Design review of the part built by this model. Coordinates are the model's own, in mm. Face numbers are marked on the shaded views. A direction names the side the tool comes from. Coordinates: 2 decimals unless noted, no trailing zeros. Order: outer loops, then holes, each group sorted by start corner. A loop starts at its lowest first (then second) coordinate and runs counter-clockwise, first axis right, second up. Notation, with made-up numbers: M 37.5,50 L 48.5,50 A23 ccw 48.5,76 Z; hole C 81.5,77 d7. An arc over 180 degrees is marked long. Answer as a JSON object with one key per item and string values.
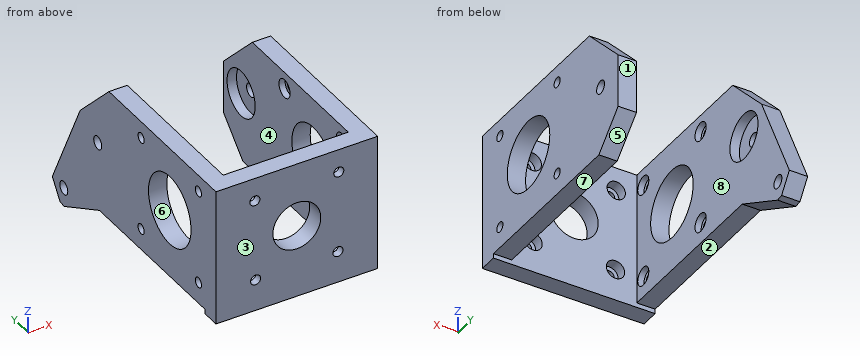
from build123d import *

# Parameters (mm, degrees)
EXTRUDE_1_DEPTH     = 64
SKETCH_2_R          = 7.85
SKETCH_2_R_2        = 1.65
CUT_EXTRUDE_1_DEPTH = 20
SKETCH_3_R          = 3
CUT_EXTRUDE_2_DEPTH = 3.5
CUT_EXTRUDE_3_DEPTH = 111.938045773
SKETCH_5_R          = 11.5
SKETCH_5_R_2        = 1.65
SKETCH_5_R_3        = 2.15
CUT_EXTRUDE_4_DEPTH = 104.981969591
SKETCH_6_R          = 7.6
CUT_EXTRUDE_5_DEPTH = 3.1
CUT_EXTRUDE_START   = -3.1
SKETCH_7_R          = 7.6
CUT_EXTRUDE_6_DEPTH = 3.1
SKETCH_10_R         = 2.15
EXTRUDE_3_DEPTH     = 6
SKETCH_11_R         = 3
CUT_EXTRUDE_7_DEPTH = 2
CUT_EXTRUDE_START_2 = -2
SKETCH_12_R         = 3
CUT_EXTRUDE_8_DEPTH = 2


with BuildPart() as part:
    # 草图1 → 凸台-拉伸1 (new body)
    with BuildSketch(Plane.XY):
        Polygon((-20.5, 73.5), (-26.5, 73.5), (-26.5, 0), (26.5, 0), (26.5, 73.5), (20.5, 73.5), (20.5, 6), (-20.5, 6), align=None)
    extrude(amount=EXTRUDE_1_DEPTH)

    # 草图2 → 切除-拉伸1 (cut)
    with BuildSketch(Plane(origin=(0, 6, 0), x_dir=(1, 0, 0), z_dir=(0, 1, 0))):
        with Locations(Location((0, -30, 0), (0, 0, 180))):
            Circle(SKETCH_2_R)
        with Locations(Location((-13.5, -16.374856692, 0), (0, 0, 180))):
            Circle(SKETCH_2_R_2)
        with Locations(Location((-13.749126603, -43.373707333, 0), (0, 0, 180))):
            Circle(SKETCH_2_R_2)
        with Locations(Location((13.749126603, -43.373707333, 0), (0, 0, 180))):
            Circle(SKETCH_2_R_2)
        with Locations(Location((13.5, -16.374856692, 0), (0, 0, 180))):
            Circle(SKETCH_2_R_2)
    extrude(amount=-CUT_EXTRUDE_1_DEPTH, mode=Mode.SUBTRACT)

    # 草图3 → 切除-拉伸2 (cut)
    with BuildSketch(Plane(origin=(0, 6, 0), x_dir=(1, 0, 0), z_dir=(0, 1, 0))):
        with Locations(Location((-13.5, -16.374856692, 0), (0, 0, 180))):
            Circle(SKETCH_3_R)
        with Locations(Location((13.5, -16.374856692, 0), (0, 0, 180))):
            Circle(SKETCH_3_R)
        with Locations(Location((13.749126603, -43.373707333, 0), (0, 0, 180))):
            Circle(SKETCH_3_R)
        with Locations(Location((-13.749126603, -43.373707333, 0), (0, 0, 180))):
            Circle(SKETCH_3_R)
    extrude(amount=-CUT_EXTRUDE_2_DEPTH, mode=Mode.SUBTRACT)

    # 草图4 → 切除-拉伸3 (cut, through all)
    with BuildSketch(Plane(origin=(26.5, 0, 0), x_dir=(0, 0, -1), z_dir=(1, 0, 0))):
        Polygon((-64, 0), (-51, 0), (-51, 57.922560455), (-35.422560455, 73.5), (-64, 73.5), align=None)
        Polygon((-6, 6), (-6, 0), (0, 0), (0, 73.5), (-17.922560455, 73.5), (-7.5, 63.077439545), (-7.5, 6), align=None)
    extrude(amount=-CUT_EXTRUDE_3_DEPTH, mode=Mode.SUBTRACT)

    # 草图5 → 切除-拉伸4 (cut, through all)
    with BuildSketch(Plane(origin=(26.5, 0, 0), x_dir=(0, 0, -1), z_dir=(1, 0, 0))):
        with Locations(Location((-30, 25, 0), (0, 0, 90))):
            Circle(SKETCH_5_R)
        with Locations(Location((-45.5, 9.5, 0), (0, 0, 90))):
            Circle(SKETCH_5_R_2)
        with Locations(Location((-14.5, 9.5, 0), (0, 0, 90))):
            Circle(SKETCH_5_R_2)
        with Locations(Location((-14.5, 40.5, 0), (0, 0, 90))):
            Circle(SKETCH_5_R_2)
        with Locations(Location((-45.5, 40.5, 0), (0, 0, 90))):
            Circle(SKETCH_5_R_2)
        with Locations(Location((-30, 64, 0), (0, 0, 90))):
            Circle(SKETCH_5_R_3)
    extrude(amount=-CUT_EXTRUDE_4_DEPTH, mode=Mode.SUBTRACT)

    # 草图6 → 切除-拉伸5 (cut)
    with BuildSketch(Plane(origin=(-20.5, 0, 0), x_dir=(0, 0, -1), z_dir=(1, 0, 0))):
        with Locations(Location((-30, 64, 0), (0, 0, 90))):
            Circle(SKETCH_6_R)
    extrude(amount=-CUT_EXTRUDE_5_DEPTH, mode=Mode.SUBTRACT)

    # 草图7 → 切除-拉伸6 (cut)
    with BuildSketch(Plane.ZY.offset(-20.5).offset(CUT_EXTRUDE_START)):
        with Locations(Location((30, 64, 0), (0, 0, 90))):
            Circle(SKETCH_7_R)
    extrude(amount=CUT_EXTRUDE_6_DEPTH, mode=Mode.SUBTRACT)

    # 草图10 → 凸台-拉伸3 (add)
    with BuildSketch(Plane.ZY.offset(26.5)):
        Polygon((35.422560455, 73.5), (4.042079148, 88.554140582), (-2.082502765, 84.366551206), (-2.369521453, 82.13565887), (7.5, 63.077439545), (17.922560455, 73.5), align=None)
        with Locations(Location((3.787134583, 82.354445963, 0), (0, 0, 270))):
            Circle(SKETCH_10_R, mode=Mode.SUBTRACT)
    extrude(amount=-EXTRUDE_3_DEPTH)

    # 草图11 → 切除-拉伸7 (cut)
    with BuildSketch(Plane(origin=(-20.5, 0, 0), x_dir=(0, 0, -1), z_dir=(1, 0, 0))):
        with Locations(Location((-45.5, 40.5, 0), (0, 0, 90))):
            Circle(SKETCH_11_R)
        with Locations(Location((-14.5, 40.5, 0), (0, 0, 90))):
            Circle(SKETCH_11_R)
        with Locations(Location((-45.5, 9.5, 0), (0, 0, 90))):
            Circle(SKETCH_11_R)
        with Locations(Location((-14.5, 9.5, 0), (0, 0, 90))):
            Circle(SKETCH_11_R)
    extrude(amount=-CUT_EXTRUDE_7_DEPTH, mode=Mode.SUBTRACT)

    # 草图12 → 切除-拉伸8 (cut)
    with BuildSketch(Plane.ZY.offset(-20.5).offset(CUT_EXTRUDE_START_2)):
        with Locations(Location((14.5, 40.5, 0), (0, 0, 90))):
            Circle(SKETCH_12_R)
        with Locations(Location((45.5, 40.5, 0), (0, 0, 90))):
            Circle(SKETCH_12_R)
        with Locations(Location((45.5, 9.5, 0), (0, 0, 90))):
            Circle(SKETCH_12_R)
        with Locations(Location((14.5, 9.5, 0), (0, 0, 90))):
            Circle(SKETCH_12_R)
    extrude(amount=CUT_EXTRUDE_8_DEPTH, mode=Mode.SUBTRACT)


solid = part.part
1) Add section C-C (y = 18). State the section outline as (x, z) points, and give its area (3 significant figures).
Taken from the geometry:
{"outline": "M -26.5,7.5 L -20.5,7.5 L -20.5,20.88 L -26.5,20.88 Z; M -26.5,39.12 L -20.5,39.12 L -20.5,51 L -26.5,51 Z; M 20.5,7.5 L 26.5,7.5 L 26.5,20.88 L 20.5,20.88 Z; M 20.5,39.12 L 26.5,39.12 L 26.5,51 L 20.5,51 Z", "area": "303 mm2"}
2) Add section D-D (x = 5). State the section outline as (y, z) points.
Taken from the geometry:
{"outline": "M 0,6 L 6,6 L 6,23.95 L 0,23.95 Z; M 0,36.05 L 6,36.05 L 6,51 L 0,51 Z"}
3) Add section A-A (z = 23.5). State the section outline as (x, y) points, and give its area (3 significant figures).
Taken from the geometry:
{"outline": "M -26.5,0 L -4.4,0 L -4.4,6 L -20.5,6 L -20.5,15.51 L -26.5,15.51 Z; M -26.5,34.49 L -20.5,34.49 L -20.5,60.06 L -23.6,60.06 L -23.6,67.94 L -20.5,67.94 L -20.5,79.22 L -26.5,79.22 Z; M 4.4,0 L 26.5,0 L 26.5,15.51 L 20.5,15.51 L 20.5,6 L 4.4,6 Z; M 20.5,34.49 L 26.5,34.49 L 26.5,73.5 L 20.5,73.5 L 20.5,67.94 L 23.6,67.94 L 23.6,60.06 L 20.5,60.06 Z", "area": "833 mm2"}
4) Insertion check: pin 1 Ø6.5 at (x, y) = (-24.5, 42.5) entering from -Z; pin 2 Ø1.8 at (y, z) = (39.5, 14.5) entering from +X; pin 3 Ø5.5 at (x, z) = (13.75, 43.37) entering from +Y; pin 4 Ø6.5 at (x, y) = (-9.5, 4.5) entering from -Z. Each pin has a flat end and moves straight along its axis. Give the tip position at first contact, or say it passes through.
Taken from the geometry:
{"pin 1": "stops at z = 7.5", "pin 2": "stops at x = 26.5", "pin 3": "stops at y = 2.5", "pin 4": "stops at z = 6"}
5) Add section B-B (x = 13.5). State the section outline as (y, z) points.
Taken from the geometry:
{"outline": "M 0,6 L 6,6 L 6,13.37 L 2.5,13.37 L 2.5,14.72 L 0,14.72 Z; M 0,18.02 L 2.5,18.02 L 2.5,19.37 L 6,19.37 L 6,40.38 L 2.5,40.38 L 2.5,41.74 L 0,41.74 Z; M 0,45 L 2.5,45 L 2.5,46.36 L 6,46.36 L 6,51 L 0,51 Z"}
6) Tool access review of the marked faces 1, 2, 3, 4 and 5: name each direction out of +Z, -Z, +X, -X, +Y, -Y from which nothing blocks a thin tool from reaching the whole face with its end or side.
Taken from the geometry:
{"face 1": "+Z, -Z, +X, +Y", "face 2": "-Z, +X, -X", "face 3": "+Z, -Z, +X, -X, -Y", "face 4": "+Z, -Z, +Y", "face 5": "-Z, +X, +Y"}
7) Mouldability with a two-part tool opening along Z and no side actions: class the marked faces 6, 7 and 8 as released by +Z, released by -Z, zero draft, split by the parting line, or undercut.
Taken from the geometry:
{"face 6": "undercut", "face 7": "released by -Z", "face 8": "zero draft"}
8) To check wall thickness, follow L1, parallel to Z at x = -24.1, y = 40.5; L2, parallel to X at y = 14.5, z = 46; L3, parallel to Z at x = 13.5, y = 1.8. State the ranges of each line that lie inside material, in increasing order.
Taken from the geometry:
{"L1": "z = 7.5 to 12.85, 16.15 to 43.85, 47.15 to 51", "L2": "x = -26.5 to -20.5, 20.5 to 26.5", "L3": "z = 6 to 14.72, 18.02 to 41.74, 45 to 51"}
